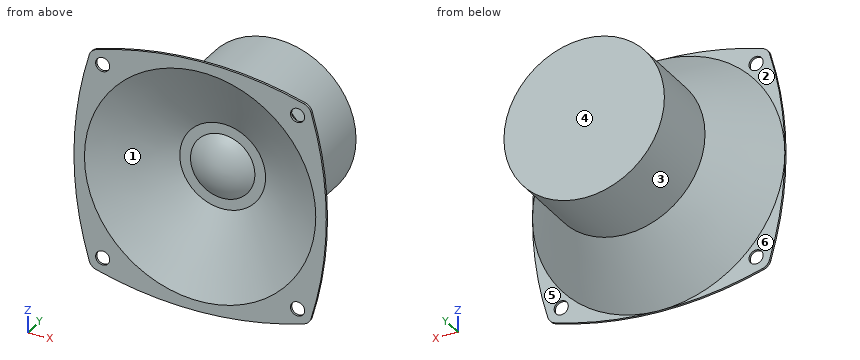
```python
from build123d import *

# Parameters (mm, degrees)
F0_R     = 24.257
F1_DEPTH = 22.86
F2_R     = 24.257
F3_DEPTH = 19.05
F3_TAPER = -36.1
F5_DEPTH = 0.6858
F6_R     = 34.97349893
F7_DEPTH = 12.7
F7_TAPER = 60
F8_R     = 2.1336
F9_DEPTH = 42.5968


with BuildPart() as f1:
    # F0 (on Front) → F1 (new body)
    with BuildSketch(Plane.XZ):
        Circle(F0_R)
    extrude(amount=F1_DEPTH)

    # F2 (on face) → F3 (join)
    with BuildSketch(Plane.XZ.offset(22.86)):
        Circle(F2_R)
    extrude(amount=F3_DEPTH, taper=F3_TAPER)

    # F4 (on face) → F5 (join)
    with BuildSketch(Plane.XZ.offset(41.91)):
        with BuildLine():
            ThreePointArc((33.5223912747, 31.3980251207), (32.7273744523, 32.7273744523), (31.3980251207, 33.5223912747))
            ThreePointArc((31.3980251207, 33.5223912747), (0, 38.14849893), (-31.3980251207, 33.5223912747))
            ThreePointArc((-31.3980251207, 33.5223912747), (-32.7273744523, 32.7273744523), (-33.5223912747, 31.3980251207))
            ThreePointArc((-33.5223912747, 31.3980251207), (-38.14849893, 0), (-33.5223912747, -31.3980251207))
            ThreePointArc((-33.5223912747, -31.3980251207), (-32.7273744523, -32.7273744523), (-31.3980251207, -33.5223912747))
            ThreePointArc((-31.3980251207, -33.5223912747), (0, -38.14849893), (31.3980251207, -33.5223912747))
            ThreePointArc((31.3980251207, -33.5223912747), (32.7273744523, -32.7273744523), (33.5223912747, -31.3980251207))
            ThreePointArc((33.5223912747, -31.3980251207), (38.14849893, 0), (33.5223912747, 31.3980251207))
        make_face()
    extrude(amount=F5_DEPTH)

    # F6 (on face) → F7 (cut)
    with BuildSketch(Plane.XZ.offset(42.5958)):
        Circle(F6_R)
    extrude(amount=-F7_DEPTH, taper=F7_TAPER, mode=Mode.SUBTRACT)

    # F8 (on face) → F9 (cut, through all)
    with BuildSketch(Plane.XZ.offset(42.5958)):
        with Locations((-29.464, 29.464)):
            Circle(F8_R)
        with Locations((29.464, 29.464)):
            Circle(F8_R)
        with Locations((-29.464, -29.464)):
            Circle(F8_R)
        with Locations((29.464, -29.464)):
            Circle(F8_R)
    extrude(amount=-F9_DEPTH, mode=Mode.SUBTRACT)

    # F10 (on Top) → F11 (revolve)
    with BuildSketch(Plane.XY):
        with BuildLine():
            Line((0, -20.0114808977), (0, -33.8875725865))
            ThreePointArc((0, -33.8875725865), (5.9030029242, -32.5693659519), (10.6844540753, -28.8652011141))
            Line((10.6844540753, -28.8652011141), (0, -20.0114808977))
        make_face()
    revolve(axis=Axis((0, -26.9495267421, 0), (0, 1, 0)))


solid = f1.part
```
Model file for the job. Use its own axes, mm. Face numbers are marked on the shaded views. A direction names the side the tool comes from. Coordinates: 2 decimals unless noted, no trailing zeros. Write each loop counter-clockwise with the first axis right and the second up, starting at its lowest first coordinate (ties: lowest second). Pieces come first, ordered by that corner, then holes. Notation, with made-up numbers: (-28.5, 60.25) - (16.5, 60.25) arc R17 ccw to (16.5, 65.25) - close; hole circle Ø8 at (-27, 88). An arc over 180 degrees is marked (long way). One line per question, with ' | ' between items. Start each with the question number.
Q1. Pin check, flat tips, straight feed: pin 1 (6 mm diameter, centred on y = -35.5, z = 18.5, fed in from -X); pin 2 (2 mm diameter, centred on x = -12, y = -14.5, fed in from +Z); pin 3 (2 mm diameter, centred on x = 13, z = -22.5, fed in from -Y). Stop position of each tip, or through.
Q2. 3-axis set-ups, long thin cutter, end or side, ignore diameter. For the marked faces 4, 5 and 6: which of +Z, -Z, +X, -X, +Y, -Y reach the whole face in a straight line?
Q3. Cut at A-A, the plane y = -36. List the corners of the cut face in (x, z).
Q4. Cut at B-B, the plane y = -12.5. List the corners of the cut face in (x, z).
Q5. Drill centre lines: line 1 (Y direction, x = 34.5, z = -25); line 2 (Z direction, x = 0.5, y = -16.5); line 3 (X direction, y = -16, z = -1). Where is each one in solid material? Low to high. Write a range as [from, to].
Q6. Pull direction Z, two halves, no side cores. Call the marked faces 1, 2 and 3: pulls with the +Z half, pulls with the -Z half, needs draft (parallel to the pull), parting line crosses it, or undercut.
Answer below:
1) pin 1: x = -31.02 | pin 2: z = 21.62 | pin 3: y = -37.98
2) face 4: +Z, -Z, +X, -X, +Y | face 5: -Z, +X, +Y | face 6: -Z, -X, +Y
3) outline: circle Ø67.68 at (0, 0); hole circle Ø47.1 at (0, 0)
4) outline: circle Ø48.51 at (0, 0)
5) line 1: [-42.6, -41.91] | line 2: [-24.25, 24.25] | line 3: [-24.24, 24.24]
6) face 1: undercut | face 2: needs draft | face 3: parting line crosses it
